For this review, use the dimensioned drawing (mm, ordinates from the lowest corner) and the shaded views. A direction names the side the tool comes from. Coordinates: 2 decimals unless noted, no trailing zeros. Write each loop counter-clockwise with the first axis right and the second up, starting at its lowest first coordinate (ties: lowest second). Pieces come first, ordered by that corner, then holes. Notation, with made-up numbers: (53, 60) - (112, 60) arc R29 ccw to (112, 96) - close; hole circle Ø2 at (21.25, 41). An arc over 180 degrees is marked (long way). Answer as a JSON object with one key per item and string values.
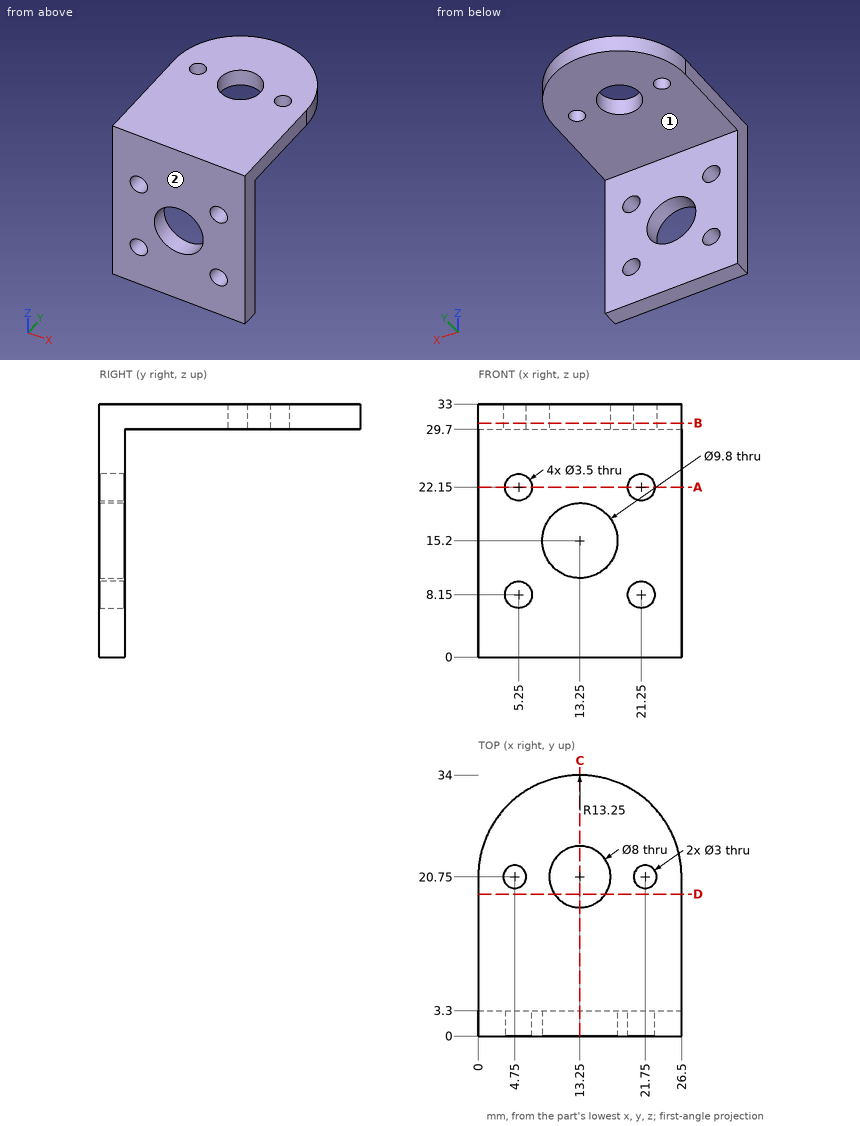
(1) Take a section at C-C, the plane x = 13.25. Write out the cut boundary in (y, z), and give its area (3 significant figures).
Solved:
{"outline": "(0, 0) - (3.3, 0) - (3.3, 10.3) - (0, 10.3) - close; (0, 20.1) - (3.3, 20.1) - (3.3, 29.7) - (16.75, 29.7) - (16.75, 33) - (0, 33) - close; (24.75, 29.7) - (34, 29.7) - (34, 33) - (24.75, 33) - close", "area": "151 mm^2"}
(2) Take a section at B-B, the plane z = 30.5. Write out the cut boundary in (x, y).
Solved:
{"outline": "(0, 0) - (26.5, 0) - (26.5, 20.75) arc R13.25 ccw to (0, 20.75) - close; hole circle Ø3 at (4.75, 20.75); hole circle Ø8 at (13.25, 20.75); hole circle Ø3 at (21.75, 20.75)"}
(3) Tool access review of the marked faces 1 and 2: name each direction out of +Z, -Z, +X, -X, +Y, -Y from which nothing blocks a thin tool from reaching the whole face with its end or side.
Solved:
{"face 1": "-Z, +X, -X, +Y", "face 2": "+Z, -Z, +X, -X, -Y"}
(4) For pin 1 (4 mm diameter, centred on x = 5.25, z = 8.15, fed in from +Y); pin 2 (4 mm diameter, centred on y = 5.5, z = 4, fed in from -X); pin 3 (10 mm diameter, centred on x = 19.5, y = 19, fed in from -Z), all flat-tipped, find the tip position at first contact; note any pin that passes through.
Solved:
{"pin 1": "stops at y = 3.3", "pin 2": "passes through", "pin 3": "stops at z = 29.7"}
(5) Take a section at D-D, the plane y = 18.5. Write out the cut boundary in (x, z), and give its area (3 significant figures).
Solved:
{"outline": "(0, 29.7) - (9.94, 29.7) - (9.94, 33) - (0, 33) - close; (16.56, 29.7) - (26.5, 29.7) - (26.5, 33) - (16.56, 33) - close", "area": "65.6 mm^2"}
(6) Take a section at A-A, the plane z = 22.15. Write out the cut boundary in (x, y).
Solved:
{"outline": "(0, 0) - (3.5, 0) - (3.5, 3.3) - (0, 3.3) - close; (7, 0) - (19.5, 0) - (19.5, 3.3) - (7, 3.3) - close; (23, 0) - (26.5, 0) - (26.5, 3.3) - (23, 3.3) - close"}
(7) To check wall thickness, follow line 1 (X direction, y = 1, z = 8); line 2 (Z direction, x = 13.25, y = 1.05); line 3 (Z direction, x = 5.5, y = 1). State the ranges of each line that lie inside material, in increasing order. Write a range as from..to.
Solved:
{"line 1": "x = 0..3.51, 6.99..19.51, 22.99..26.5", "line 2": "z = 0..10.3, 20.1..33", "line 3": "z = 0..6.42, 9.88..20.42, 23.88..33"}
